from build123d import *

# Parameters (mm, degrees)
F1_DEPTH = 15
F3_START = 10
F2_R     = 14
F3_DEPTH = 15


with BuildPart() as f1:
    # F0 (on Front) → F1 (new body)
    with BuildSketch(Plane.XZ):
        with BuildLine():
            Line((-24.8721406347, 47.4748029292), (-19.9908943662, -0.603442158))
            Line((-19.9908943662, -0.603442158), (-19.7042578352, -3.4266927442))
            ThreePointArc((-19.7042578352, -3.4266927442), (-1.1601406694, -19.966323488), (19.1747802681, -5.6857542744))
            Line((19.1747802681, -5.6857542744), (19.8706965994, 2.2705542616))
            Line((19.8706965994, 2.2705542616), (21.7154896457, 23.361800439))
            ThreePointArc((21.7154896457, 23.361800439), (23.1184617772, 26.4186682546), (26.1405225938, 27.895123491))
            Line((26.1405225938, 27.895123491), (89.6744252597, 35.0035337133))
            ThreePointArc((89.6744252597, 35.0035337133), (104.9669737345, 49.0051647211), (91.6621115435, 64.9076284236))
            Line((91.6621115435, 64.9076284236), (27.4153419388, 71.2848644166))
            ThreePointArc((27.4153419388, 71.2848644166), (23.7872845646, 72.9910681825), (22.0437681238, 76.6013426904))
            Line((22.0437681238, 76.6013426904), (15.089959345, 140))
            Line((15.089959345, 140), (15, 140))
            ThreePointArc((15, 140), (14.9776275535, 140.8189461935), (14.910576951, 141.6354494764))
            ThreePointArc((14.910576951, 141.6354494764), (0.0042894025, 154.9999993867), (-14.9096391656, 141.6439768707))
            Line((-14.9096391656, 141.6439768707), (-24.4285254093, 55.3148066248))
            ThreePointArc((-24.4285254093, 55.3148066248), (-24.960074773, 51.4123310642), (-24.8721406347, 47.4748029292))
        make_face()
        with BuildLine():
            ThreePointArc((10, 0), (-7.0710678119, -7.0710678119), (0, 10))
            ThreePointArc((0, 10), (7.0710678119, 7.0710678119), (10, 0))
        make_face(mode=Mode.SUBTRACT)
        with BuildLine():
            ThreePointArc((0, 30), (-20, 50), (0, 70))
            ThreePointArc((0, 70), (14.1421356237, 64.1421356237), (20, 50))
            ThreePointArc((20, 50), (14.1421356237, 35.8578643763), (0, 30))
        make_face(mode=Mode.SUBTRACT)
        with BuildLine():
            ThreePointArc((97.5, 50), (90, 42.5), (82.5, 50))
            ThreePointArc((82.5, 50), (90, 57.5), (97.5, 50))
        make_face(mode=Mode.SUBTRACT)
        with BuildLine():
            ThreePointArc((0, 132.5), (-5.3033008589, 145.3033008589), (7.5, 140))
            ThreePointArc((7.5, 140), (5.3033008589, 134.6966991411), (0, 132.5))
        make_face(mode=Mode.SUBTRACT)
    extrude(amount=F1_DEPTH)

    # F2 (on Front) → F3 (cut)
    with BuildSketch(Plane.XZ.offset(F3_START)):
        Circle(F2_R)
    extrude(amount=F3_DEPTH, mode=Mode.SUBTRACT)


solid = f1.part
The listing builds one solid part. Answer for the finished solid, in the listing's coordinates (mm). A direction names the side the tool comes from. Coordinates: 2 decimals unless noted, no trailing zeros. Loops run counter-clockwise (first coordinate to the right, second up) from the corner with the lowest first, then second, coordinate; pieces in that order, holes last. Notation, with made-up numbers: M -25,53 L 34,53 A21 cw 34,63 Z; hole C 87.5,-6 d1. An arc over 180 degrees is marked long. Answer in a Markdown table with one row per item.
1) Determine the mould class of faces 3 (the cylindrical face through (-0.976, -7.395, 132.564)), 4 (the flat face through (20, 0, 55)), 5 (the flat face through (59.99, -7.4, 68.05)) for opening direction Z: released by +Z, released by -Z, zero draft, split by the parting line, or undercut.
Answers below:
| item | result |
|---|---|
| face 3 | undercut |
| face 4 | zero draft |
| face 5 | released by +Z |
2) Find section A-A (y = -7.5). Determine the outline of the cut face in (x, z).
Answers below:
| item | result |
|---|---|
| outline | M -24.87,47.47 L -19.7,-3.43 A20 ccw 19.17,-5.69 L 21.72,23.36 A5 cw 26.14,27.9 L 89.67,35 A15 ccw 91.66,64.91 L 27.42,71.28 A6 cw 22.04,76.6 L 15.09,140 L 15,140 A15 ccw -14.91,141.64 L -24.43,55.31 A25 ccw Z; hole C 0,50 d40; hole C 0,0 d20; hole C 0,140 d15; hole C 90,50 d15 |
3) Find section B-B (x = 37.5). Determine the outline of the cut face in (y, z), then the cut area to 3 significant figures.
Answers below:
| item | result |
|---|---|
| outline | M -15,29.17 L 0,29.17 L 0,70.28 L -15,70.28 Z |
| area | 617 mm^2 |
4) Which of the six approach directions +Z, -Z, +X, -X, +Y, -Y give full straight-line access (tool end or side, diameter ignored) to faces 1 (the cylindrical face through (12.932, -12.465, -5.362)), 2 (the cylindrical face through (23.83, -7.4, 72.95))?
Answers below:
| item | result |
|---|---|
| face 1 | -Y |
| face 2 | +Z, +X, +Y, -Y |
5) Find the intervals of material crossed by probe 1 along Z at (x, y) = (0, -3.5); probe 2 along X at (y, z) = (-12.6, 0); probe 3 along X at (y, z) = (-4, 5), in increasing order.
Answers below:
| item | result |
|---|---|
| probe 1 | -20 to -10, 10 to 30, 70 to 132.5, 147.5 to 155 |
| probe 2 | -20.05 to -14, 14 to 19.67 |
| probe 3 | -20.56 to -8.66, 8.66 to 20.11 |
6) Given pin 1 (22.5 mm diameter, centred on x = 2.5, z = 1, fed in from -Y); pin 2 (2 mm diameter, centred on y = -3, z = 99.5, fed in from -X); pin 3 (6 mm diameter, centred on y = -5, z = 110.5, fed in from +X); pin 4 (17 mm diameter, centred on x = 90, z = 50, fed in from -Y), each flat-ended and moving along its own axis, determine where each tip first touches the part or whether it passes through.
Answers below:
| item | result |
|---|---|
| pin 1 | y = -10 |
| pin 2 | x = -19.67 |
| pin 3 | x = 18.65 |
| pin 4 | y = -15 |
7) Find section C-C (z = 79.5). Determine the outline of the cut face in (x, y), then the cut area to 3 significant figures.
Answers below:
| item | result |
|---|---|
| outline | M -21.76,-15 L 21.73,-15 L 21.73,0 L -21.76,0 Z |
| area | 652 mm^2 |
